Geometry check sheet. Reference: the model listing, model coordinates, mm. A direction names the side the tool comes from. Give positions to 0.01 mm unless a question says otherwise; leave off trailing zeros. Order: outer loops, then holes, each group sorted by start corner. A loop starts at its lowest first (then second) coordinate and runs counter-clockwise, first axis right, second up.
from build123d import *

# Parameters (mm, degrees)
F0_R     = 1.8
F1_DEPTH = 3
F2_R     = 2.49999
F3_W     = 15.2
F3_H     = 29.6
F4_DEPTH = 3


# Not quite as in the source:
# - a fillet or chamfer is up to 0.001 mm smaller than in the source, because OpenCascade refuses the exact size


with BuildPart() as f1:
    # F0 (on Top) → F1 (new body)
    with BuildSketch(Plane.XY):
        Polygon((-34.8, 9.6), (-34.8, 0), (34.8, 0), (34.8, 9.6), (29.8, 9.6), (29.8, 39.6), (-29.8, 39.6), (-29.8, 9.6), align=None)
        with Locations((-30, 4.8)):
            Circle(F0_R, mode=Mode.SUBTRACT)
        with Locations((30, 4.8)):
            Circle(F0_R, mode=Mode.SUBTRACT)
        with Locations((-25, 19.8)):
            Circle(F0_R, mode=Mode.SUBTRACT)
        with Locations((-25, 34.8)):
            Circle(F0_R, mode=Mode.SUBTRACT)
        with Locations((25, 19.8)):
            Circle(F0_R, mode=Mode.SUBTRACT)
        with Locations((25, 34.8)):
            Circle(F0_R, mode=Mode.SUBTRACT)
    extrude(amount=F1_DEPTH)

    # F2 (radius 2.5 in the source; OpenCascade refuses exactly that, so slightly less here)
    f2_edges = [f1.edges().sort_by_distance(p)[0] for p in [
        (-34.8, 0, 1.5),
        (-34.8, 9.6, 1.5),
        (-29.8, 9.6, 1.5),
        (34.8, 0, 1.5),
        (29.8, 9.6, 1.5),
        (34.8, 9.6, 1.5),
        (29.8, 39.6, 1.5),
        (-29.8, 39.6, 1.5),
    ]]
    fillet(f2_edges, radius=F2_R)

    # F3 (on face) → F4 (cut, through all)
    with BuildSketch(Plane(origin=(0, 0, 0), x_dir=(1, 0, 0), z_dir=(0, 0, -1))):
        with Locations((10.6, -19.8)):
            Rectangle(F3_W, F3_H)
        with Locations((-10.6, -19.8)):
            Rectangle(F3_W, F3_H)
    extrude(amount=-F4_DEPTH, mode=Mode.SUBTRACT)


solid = f1.part
Item 1: Scan lines: L1, parallel to X at y = 12, z = 0.7; L2, parallel to Y at x = -25, z = 1.45; L3, parallel to Y at x = -14.5, z = 0.2. Record each from-to range of solid material in increasing order.
Reported:
L1: x = -29.8 to -18.2, -3 to 3, 18.2 to 29.8
L2: y = 0 to 18, 21.6 to 33, 36.6 to 39.6
L3: y = 0 to 5, 34.6 to 39.6
Item 2: Set-up check for faces 1 (the cylindrical face through (34.048, 0.713, 1.521)), 2 (the flat face through (-29.8, 25, 1)), 3 (the flat face through (-3, 20, 1)), 4 (the flat face through (29.8, 24, 1)), 5 (the flat face through (0, 0, 1)): record each of +Z, -Z, +X, -X, +Y, -Y from which the full face is reachable in a straight line by a thin tool's end or side.
Reported:
face 1: +Z, -Z, +X, -Y
face 2: +Z, -Z, -X, +Y
face 3: +Z, -Z
face 4: +Z, -Z, +X, +Y
face 5: +Z, -Z, +X, -X, -Y
Item 3: Sectioned sample at C-C (z = 1.4). Give the number of separate pieces and of enclosed holes in the cut face, and give its area (3 significant figures).
Reported:
separate pieces: 1
enclosed holes: 8
area: 1,490 mm2
Item 4: Gauge pin test, flat ends, axial feed: pin 1 (0.9 mm diameter, centred on y = 24, z = 2, fed in from +X); pin 2 (0.9 mm diameter, centred on y = 26, z = 1.5, fed in from -X); pin 3 (2 mm diameter, centred on x = 25, y = 19.8, fed in from -Z). Record the tip position at first contact, or that the pin passes through.
Reported:
pin 1: stops at x = 29.8
pin 2: stops at x = -29.8
pin 3: passes through
Item 5: Sectioned sample at A-A (y = 26.5). Enter the section's corners in (x, z).
Reported:
outline: (-29.8, 0) - (-18.2, 0) - (-18.2, 3) - (-29.8, 3) - close; (-3, 0) - (3, 0) - (3, 3) - (-3, 3) - close; (18.2, 0) - (29.8, 0) - (29.8, 3) - (18.2, 3) - close
Item 6: Sectioned sample at B-B (x = -25). Enter the section's corners in (y, z), and give its area (3 significant figures).
Reported:
outline: (0, 0) - (18, 0) - (18, 3) - (0, 3) - close; (21.6, 0) - (33, 0) - (33, 3) - (21.6, 3) - close; (36.6, 0) - (39.6, 0) - (39.6, 3) - (36.6, 3) - close
area: 97.2 mm2
Item 7: Draft check along X on faces 6 (the flat face through (34.8, 5, 1)), 7 (the cylindrical face through (-30.552, 10.313, 1.521)), 8 (the cylindrical face through (26.717, 35.341, 1.479)). Enter one of: released by +X, released by -X, zero draft, split by the parting line, or undercut.
Reported:
face 6: released by +X
face 7: released by -X
face 8: undercut
